Could you check a few things on this model? Use its own coordinates, in mm. A direction names the side the tool comes from. Coordinates: 2 decimals unless noted, no trailing zeros. Order: outer loops, then holes, each group sorted by start corner. A loop starts at its lowest first (then second) coordinate and runs counter-clockwise, first axis right, second up. Notation, with made-up numbers: (-12.5, 42.5) - (29.5, 42.5) arc R19 cw to (29.5, 70.5) - close; hole circle Ø9 at (13, 1.5). An arc over 180 degrees is marked (long way). Answer as a JSON object with one key per item and string values. Group by question number.
(1) Which directions (+Z, -Z, +X, -X, +Y, -Y) give clear straight access to the entire face, cutting with the end or side of a thin tool? Please do faces 1 (the flat face through (-9.2, 29.6, -3.7)), 2 (the flat face through (-4.5, 29.6, -6)), 3 (the flat face through (-10, 30, 7)), 4 (the flat face through (0, 30, -4.5)), 5 (the flat face through (3.8, 29.6, 9.3)).
(2) Imagine slicing it at A-A, the plane x = 0. Write out the boundary of the cut face in (y, z), and give its area (3 significant figures).
(3) Will these pins go through, and if not, where does the flat tip stop? P1, Ø5, axis at y = 32.5, z = 1.5, coming from the -X side; P2, Ø6.5, axis at y = 44.5, z = -0.5, coming from the -X side; P3, Ø5, axis at y = 22.5, z = 1.5, coming from the +X side.
(4) We'd pull the mould along X, two halves only. Please class faces 6 (the flat face through (-3.8, 29.6, -9.3)), 7 (the flat face through (10, 30, 7)), 8 (the flat face through (-4.5, 30, 0)), 9 (the flat face through (-7, 30, -10)): pulls with the +X half, pulls with the -X half, needs draft (parallel to the pull), parting line crosses it, or undercut.
(5) Please list where these lines run through material, in increasing order: probe 1 along X at (y, z) = (17, 0); probe 2 along X at (y, z) = (24.5, -3.75); probe 3 along X at (y, z) = (35.5, -5).
(6) Imagine slicing it at B-B, the plane z = 0. Write out the boundary of the cut face in (x, y), and give its area (3 significant figures).
from build123d import *

# Parameters (mm, degrees)
BOSS_EXTRUDE2_DEPTH = 60
SKETCH1_3_R         = 2.75
CUT_EXTRUDE4_DEPTH  = 80
FILLET7_R           = 0.75
FILLET8_R           = 0.5


with BuildPart() as part:
    # Sketch1 → Boss-Extrude2 (new body)
    with BuildSketch(Plane(origin=(0, 0, 0), x_dir=(1, 0, 0), z_dir=(0, 1, 0))):
        Polygon((-3, 4.5), (3, 4.5), (6, 7.5), (6, 8.5), (3, 8.5), (4.5, 10), (10, 10), (10, 4.5), (8.5, 3), (8.5, 6), (7.5, 6), (4.5, 3), (4.5, -3), (7.5, -6), (8.5, -6), (8.5, -3), (10, -4.5), (10, -10), (4.5, -10), (3, -8.5), (6, -8.5), (6, -7.5), (3, -4.5), (-3, -4.5), (-6, -7.5), (-6, -8.5), (-3, -8.5), (-4.5, -10), (-10, -10), (-10, -4.5), (-8.5, -3), (-8.5, -6), (-7.5, -6), (-4.5, -3), (-4.5, 3), (-7.5, 6), (-8.5, 6), (-8.5, 3), (-10, 4.5), (-10, 10), (-4.5, 10), (-3, 8.5), (-6, 8.5), (-6, 7.5), align=None)
    extrude(amount=BOSS_EXTRUDE2_DEPTH)

    # Sketch1<3> → Cut-Extrude4 (cut)
    with BuildSketch(Plane(origin=(0, 0, 0), x_dir=(1, 0, 0), z_dir=(0, 1, 0))):
        Circle(SKETCH1_3_R)
    extrude(amount=CUT_EXTRUDE4_DEPTH, mode=Mode.SUBTRACT)

    # Fillet7
    fillet7_edges = [part.edges().sort_by_distance(p)[0] for p in [
        (-10, 30, -10),
        (10, 30, -10),
        (10, 30, 10),
        (-10, 30, 10),
    ]]
    fillet(fillet7_edges, radius=FILLET7_R)

    # Fillet8
    fillet8_edges = [part.edges().sort_by_distance(p)[0] for p in [
        (-6, 30, -8.5),
        (6, 30, -8.5),
        (8.5, 30, -6),
        (8.5, 30, 6),
        (6, 30, 8.5),
        (-6, 30, 8.5),
        (-8.5, 30, 6),
        (-8.5, 30, -6),
    ]]
    fillet(fillet8_edges, radius=FILLET8_R)


solid = part.part
Result set:
{
 "1": {"face 1": "-X, +Y, -Y", "face 2": "+Y, -Y", "face 3": "+Z, -Z, -X, +Y, -Y", "face 4": "-Z, +Y, -Y", "face 5": "+Z, +Y, -Y"},
 "2": {"outline": "(0, -4.5) - (60, -4.5) - (60, -2.75) - (0, -2.75) - close; (0, 2.75) - (60, 2.75) - (60, 4.5) - (0, 4.5) - close", "area": "210 mm^2"},
 "3": {"P1": "stops at x = -9.5", "P2": "stops at x = -9.25", "P3": "stops at x = 9.5"},
 "4": {"face 6": "undercut", "face 7": "pulls with the +X half", "face 8": "pulls with the -X half", "face 9": "needs draft"},
 "5": {"probe 1": "x = -4.5 to -2.75, 2.75 to 4.5", "probe 2": "x = -9.25 to -8.5, -5.25 to 5.25, 8.5 to 9.25", "probe 3": "x = -10 to -8.5, -6.5 to -3.5, 3.5 to 6.5, 8.5 to 10"},
 "6": {"outline": "(-4.5, 0) - (-2.75, 0) - (-2.75, 60) - (-4.5, 60) - close; (2.75, 0) - (4.5, 0) - (4.5, 60) - (2.75, 60) - close", "area": "210 mm^2"}
}
